Study the drawing (mm; zero at the part's minimum x, y, z) and answer. A direction names the side the tool comes from. Give positions to 0.01 mm unless a question says otherwise; leave off trailing zeros. Order: outer loops, then holes, each group sorted by start corner. A loop starts at its lowest first (then second) coordinate and runs counter-clockwise, first axis right, second up.
Item 1: Given pin 1 Ø7 at (x, y) = (39, 39) entering from -Z; pin 2 Ø5 at (x, y) = (39, 9) entering from +Z; pin 3 Ø7 at (x, y) = (9, 39) entering from +Z; pin 4 Ø4 at (x, y) = (21.5, 42.5) entering from +Z, each flat-ended and moving along its own axis, determine where each tip first touches the part or whether it passes through.
Item 2: A cutting plane is placed at A-A (x = 39). Write down the section's boundary in (y, z), plus the area to 3 significant figures.
Item 3: Which of the six approach directions +Z, -Z, +X, -X, +Y, -Y give full straight-line access (tool end or side, diameter ignored) to the marked faces 1, 2 and 3?
Item 4: The mould has two halves that part along X. Classify the marked faces 4, 5, 6 and 7: +X half, -X half, draft (parallel to the pull), parting line (faces both ways), or undercut.
Item 5: A cutting plane is placed at D-D (y = 33). Write down the section's boundary in (x, z).
Item 6: A cutting plane is placed at C-C (z = 7.5). Write down the section's boundary in (x, y).
Item 7: Find the intervals of material crossed by line 1 along X through (y, z) = (39, 7.75); line 2 along Z through (x, y) = (4, 20.5), in increasing order.
Item 8: A cutting plane is placed at B-B (y = 9). Write down the section's boundary in (x, z).
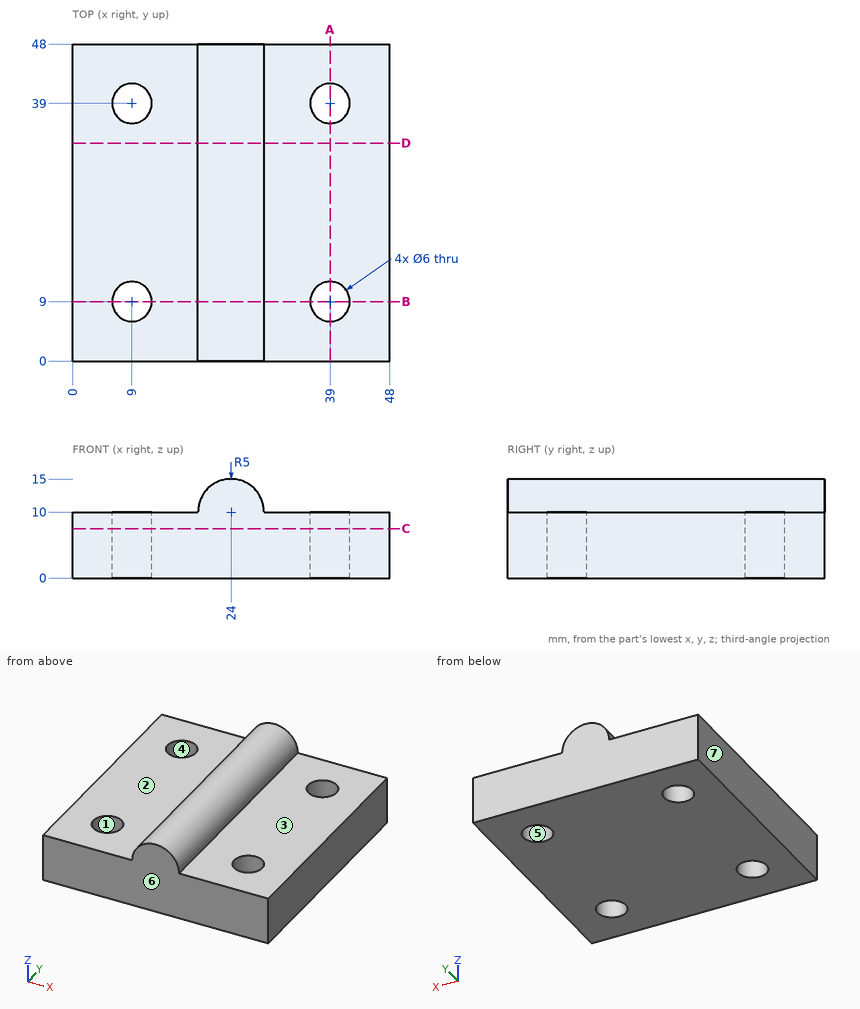
Response values:
1. pin 1: stops at z = 0
1. pin 2: passes through
1. pin 3: stops at z = 10
1. pin 4: stops at z = 14.97
2. outline: (0, 0) - (6, 0) - (6, 10) - (0, 10) - close; (12, 0) - (36, 0) - (36, 10) - (12, 10) - close; (42, 0) - (48, 0) - (48, 10) - (42, 10) - close
2. area: 360 mm2
3. face 1: +Z, -Z
3. face 2: +Z, -X, +Y, -Y
3. face 3: +Z, +X, +Y, -Y
4. face 4: undercut
4. face 5: undercut
4. face 6: draft
4. face 7: -X half
5. outline: (0, 0) - (48, 0) - (48, 10) - (29, 10) arc R5 ccw to (19, 10) - (0, 10) - close
6. outline: (0, 0) - (48, 0) - (48, 48) - (0, 48) - close; hole circle Ø6 at (9, 9); hole circle Ø6 at (9, 39); hole circle Ø6 at (39, 9); hole circle Ø6 at (39, 39)
7. line 1: x = 0 to 6, 12 to 36, 42 to 48
7. line 2: z = 0 to 10
8. outline: (0, 0) - (6, 0) - (6, 10) - (0, 10) - close; (12, 0) - (36, 0) - (36, 10) - (29, 10) arc R5 ccw to (19, 10) - (12, 10) - close; (42, 0) - (48, 0) - (48, 10) - (42, 10) - close
